from build123d import *

# Parameters (mm, degrees)
ESQUISSE1_W             = 3
ESQUISSE1_H             = 55
BOSS_EXTRU_1_DEPTH      = 2.5
ESQUISSE2_R             = 3.5
ESQUISSE2_R_2           = 2
BOSS_EXTRU_2_DEPTH      = 5
BOSS_EXTRU_3_REACH      = 57.473
BOSS_EXTRU_3_END_RADIUS = 2
ESQUISSE3_W             = 3
ESQUISSE3_H             = 5


with BuildPart() as part:
    # Esquisse1 → Boss.-Extru.1 (new, symmetric)
    with BuildSketch(Plane.XY):
        with Locations((1.5, 27.5)):
            Rectangle(ESQUISSE1_W, ESQUISSE1_H)
    extrude(amount=BOSS_EXTRU_1_DEPTH, both=True)



with BuildPart() as body_2:
    # Esquisse2 → Boss.-Extru.2 (new, symmetric)
    with BuildSketch(Plane.XY):
        with Locations((1.718667593, -5.582160954)):
            Circle(ESQUISSE2_R)
        with Locations((1.718667593, -5.582160954)):
            Circle(ESQUISSE2_R_2, mode=Mode.SUBTRACT)
    extrude(amount=BOSS_EXTRU_2_DEPTH, both=True)


with BuildPart() as part_1:
    add(part.part)

    add(body_2.part)  # Boss.-Extru.3 merges body 2
    # Boss.-Extru.3: up to this cylinder (the profile starts outside it)
    boss_extru_3_end = Plane(origin=(1.718667593, -5.582160954, 0), z_dir=(0, 0, -1)) * Cylinder(BOSS_EXTRU_3_END_RADIUS, 119.946, mode=Mode.PRIVATE)
    # Esquisse3 → Boss.-Extru.3 (add, up to the surface)
    with BuildSketch(Plane.XZ, mode=Mode.PRIVATE) as boss_extru_3_sk1:
        with Locations((1.5, 0)):
            Rectangle(ESQUISSE3_W, ESQUISSE3_H)
    boss_extru_3_tool1 = extrude(boss_extru_3_sk1.sketch, amount=BOSS_EXTRU_3_REACH, mode=Mode.PRIVATE) - boss_extru_3_end
    add(boss_extru_3_tool1.solids().sort_by_distance((1.5, 0, 0))[0])


solid = part_1.part
Source: CAD feature listing. Evaluate the final solid. Frame: model axes, mm. A direction names the side the tool comes from. Coordinates: 2 decimals unless noted, no trailing zeros. Loops run counter-clockwise (first coordinate to the right, second up) from the corner with the lowest first, then second, coordinate; pieces in that order, holes last. Notation, with made-up numbers: M 23.5,67.5 L 77.5,67.5 A11 cw 77.5,78.5 Z; hole C 52,77 d9. An arc over 180 degrees is marked long. Answer in a Markdown table with one row per item.
Q1. First-contact query: pin 1 (3 mm diameter, centred on y = 10.5, z = 3.5, fed in from -X); pin 2 (2 mm diameter, centred on y = 21.5, z = -2.5, fed in from +X); pin 3 (0.9 mm diameter, centred on x = 1, y = 39, fed in from -Z). Flat tips, straight axial feed; report the tip coordinate or a pass-through.
Answers below:
| item | result |
|---|---|
| pin 1 | stops at x = 0 |
| pin 2 | stops at x = 3 |
| pin 3 | stops at z = -2.5 |
Q2. Draft query along Y for faces 1 (the cylindrical face through (0.96, -9, 0.07)), 2 (the flat face through (1, 27, -2.5)), 3 (the flat face through (1, 55, 0)), 4 (the cylindrical face through (1.46, -3.6, -0.07)). Return one class per face: pulls with the +Y half, pulls with the -Y half, needs draft (parallel to the pull), parting line crosses it, or undercut.
Answers below:
| item | result |
|---|---|
| face 1 | parting line crosses it |
| face 2 | needs draft |
| face 3 | pulls with the +Y half |
| face 4 | undercut |
Q3. Set-up query: faces 5 (the flat face through (4, -6, -5)), 6 (the flat face through (3, 27, 0)), 7 (the flat face through (0, 27, 0)), 8 (the flat face through (4, -6, 5)), 9 (the flat face through (1, 27, 2.5)). Return all of +Z, -Z, +X, -X, +Y, -Y with unobstructed straight access to the full face (end or side cutting, diameter ignored); none if empty.
Answers below:
| item | result |
|---|---|
| face 5 | -Z, +X, -X, +Y, -Y |
| face 6 | +Z, -Z, +X, +Y |
| face 7 | +Z, -Z, -X, +Y |
| face 8 | +Z, +X, -X, +Y, -Y |
| face 9 | +Z, +X, -X, +Y |
Q4. Section B-B on z = 1.5. Return the cut outline in (x, y), plus the area to 3 significant figures.
Answers below:
| item | result |
|---|---|
| outline | M 0,-2.53 A3.5 ccw long 3,-2.33 L 3,55 L 0,55 Z; hole C 1.72,-5.58 d4 |
| area | 198 mm^2 |
Q5. Section D-D on z = 4. Return the cut outline in (x, y).
Answers below:
| item | result |
|---|---|
| outline | C 1.72,-5.58 d7; hole C 1.72,-5.58 d4 |
Q6. Ray query, probe 1 along Y at (x, z) = (1.75, 4.5); probe 2 along X at (y, z) = (47, 2.25); probe 3 along Y at (x, z) = (0.25, 0.5). Return the intervals inside material, ascending. Write a range as from..to.
Answers below:
| item | result |
|---|---|
| probe 1 | y = -9.08..-7.58, -3.58..-2.08 |
| probe 2 | x = 0..3 |
| probe 3 | y = -8.76..-6.94, -4.22..55 |
Q7. Section C-C on y = 2.5. Return the cut outline in (x, z), plus the area to 3 significant figures.
Answers below:
| item | result |
|---|---|
| outline | M 0,-2.5 L 3,-2.5 L 3,2.5 L 0,2.5 Z |
| area | 15.0 mm^2 |
Q8. Section A-A on x = 1. Return the cut outline in (y, z), plus the area to 3 significant figures.
Answers below:
| item | result |
|---|---|
| outline | M -9.01,-5 L -7.45,-5 L -7.45,5 L -9.01,5 Z; M -3.72,-5 L -2.16,-5 L -2.16,-2.5 L 55,-2.5 L 55,2.5 L -2.16,2.5 L -2.16,5 L -3.72,5 Z |
| area | 317 mm^2 |
